```python
from build123d import *

# Parameters (mm, degrees)
BOSS_EXTRUDE1_DEPTH = 20
SKETCH1_3_R         = 40
SKETCH1_3_R_2       = 25
BOSS_EXTRUDE2_DEPTH = 40
BOSS_EXTRUDE3_DEPTH = 70


with BuildPart() as part:
    # Sketch1 → Boss-Extrude1 (new body)
    with BuildSketch(Plane(origin=(0, 0, 0), x_dir=(1, 0, 0), z_dir=(0, 1, 0))):
        with BuildLine():
            ThreePointArc((-47.892857143, -57.717191847), (-25.457912439, -70.547109751), (0, -75))
            Line((0, -75), (0, -60))
            ThreePointArc((0, -60), (-60, 0), (0, 60))
            Line((0, 60), (0, 75))
            ThreePointArc((0, 75), (-25.457912439, 70.547109751), (-47.892857143, 57.717191847))
            ThreePointArc((-47.892857143, 57.717191847), (-91.104177178, 36.827906099), (-139.071428571, 38.478127898))
            ThreePointArc((-139.071428571, 38.478127898), (-118.084934144, 24.112830017), (-110, 0))
            ThreePointArc((-110, 0), (-118.084934144, -24.112830017), (-139.071428571, -38.478127898))
            ThreePointArc((-139.071428571, -38.478127898), (-91.104177178, -36.827906099), (-47.892857143, -57.717191847))
        make_face()
        with BuildLine():
            Line((0, -60), (0, -75))
            ThreePointArc((0, -75), (25.457912439, -70.547109751), (47.892857143, -57.717191847))
            ThreePointArc((47.892857143, -57.717191847), (91.104177178, -36.827906099), (139.071428571, -38.478127898))
            ThreePointArc((139.071428571, -38.478127898), (110, 0), (139.071428571, 38.478127898))
            ThreePointArc((139.071428571, 38.478127898), (91.104177178, 36.827906099), (47.892857143, 57.717191847))
            ThreePointArc((47.892857143, 57.717191847), (25.457912439, 70.547109751), (0, 75))
            Line((0, 75), (0, 60))
            ThreePointArc((0, 60), (42.426406871, 42.426406871), (60, 0))
            ThreePointArc((60, 0), (42.426406871, -42.426406871), (0, -60))
        make_face()
    extrude(amount=BOSS_EXTRUDE1_DEPTH)

    # Sketch1_3 → Boss-Extrude2 (add)
    # profile 1 of 2: a face of its own
    with BuildSketch(Plane(origin=(0, 0, 0), x_dir=(1, 0, 0), z_dir=(0, 1, 0))):
        with Locations(Location((-150, 0, 0), (0, 0, 74.144374523))):
            Circle(SKETCH1_3_R)
        with Locations(Location((-150, 0, 0), (0, 0, 270))):
            Circle(SKETCH1_3_R_2, mode=Mode.SUBTRACT)
    # profile 2 of 2: a face of its own
    with BuildSketch(Plane(origin=(0, 0, 0), x_dir=(1, 0, 0), z_dir=(0, 1, 0))):
        with Locations(Location((150, 0, 0), (0, 0, 105.855625477))):
            Circle(SKETCH1_3_R)
        with Locations(Location((150, 0, 0), (0, 0, 270))):
            Circle(SKETCH1_3_R_2, mode=Mode.SUBTRACT)
    extrude(amount=BOSS_EXTRUDE2_DEPTH)

    # Sketch1_4 → Boss-Extrude3 (add)
    with BuildSketch(Plane(origin=(0, 0, 0), x_dir=(1, 0, 0), z_dir=(0, 1, 0))):
        with BuildLine():
            ThreePointArc((0, 60), (-60, 0), (0, -60))
            Line((0, -60), (0, -50))
            ThreePointArc((0, -50), (-50, 0), (0, 50))
            Line((0, 50), (0, 60))
        make_face()
        with BuildLine():
            Line((0, -50), (0, -60))
            ThreePointArc((0, -60), (42.426406871, -42.426406871), (60, 0))
            ThreePointArc((60, 0), (42.426406871, 42.426406871), (0, 60))
            Line((0, 60), (0, 50))
            ThreePointArc((0, 50), (35.355339059, 35.355339059), (50, 0))
            ThreePointArc((50, 0), (35.355339059, -35.355339059), (0, -50))
        make_face()
    extrude(amount=BOSS_EXTRUDE3_DEPTH)


solid = part.part
```
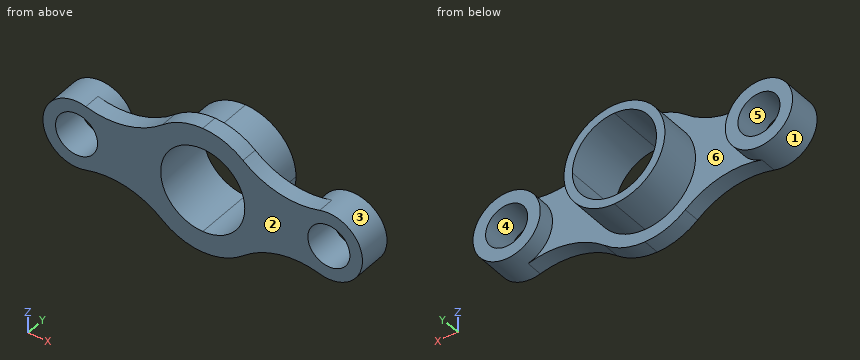
Design review of the part built by this model. Coordinates are the model's own, in mm. Face numbers are marked on the shaded views. A direction names the side the tool comes from. Coordinates: 2 decimals unless noted, no trailing zeros. Order: outer loops, then holes, each group sorted by start corner. A loop starts at its lowest first (then second) coordinate and runs counter-clockwise, first axis right, second up. Notation, with made-up numbers: M 80,23.5 L 91,23.5 A6 cw 91,28.5 Z; hole C 51.25,45.5 d4. An arc over 180 degrees is marked long. Answer as a JSON object with one key per item and string values. Group by question number.
1) Add section B-B, the plane x = -150. Write out the cut boundary in (y, z), then the cut area to 3 significant figures.
2) Add section C-C, the plane z = 10.5. Write out the cut boundary in (x, y), then the cut area to 3 significant figures.
3) Tool access review of the marked faces 1 and 2: name each direction out of +Z, -Z, +X, -X, +Y, -Y from which nothing blocks a thin tool from reaching the whole face with its end or side.
4) For pin 1 (12 mm diameter, centred on x = -87, z = 10, fed in from +Y); pin 2 (6 mm diameter, centred on y = 38, z = -7.5, fed in from +X); pin 3 (2 mm diameter, centred on x = 55.5, y = 58.5, fed in from -Z), all flat-tipped, find the tip position at first contact; note any pin that passes through.
5) Mouldability with a two-part tool opening along Z and no side actions: class the marked faces 3, 4, 5 and 6 as pulls with the +Z half, pulls with the -Z half, needs draft (parallel to the pull), parting line crosses it, or undercut.
6) Add section A-A, the plane y = 25. Write out the cut boundary in (x, z), then the cut area to 3 significant figures.
7) Wall thickness on L1, parallel to X at y = 15, z = 0; L2, parallel to Y at x = -102, z = 13.5; L3, parallel to Z at x = 22, y = 56.5: over which ranges is each line inside the solid? List them lowest first.
8) Add section D-D, the plane x = 120.5. Write out the cut boundary in (y, z), then the cut area to 3 significant figures.
Computed values:
{
 "1": {"outline": "M 0,-40 L 40,-40 L 40,-25 L 0,-25 Z; M 0,25 L 40,25 L 40,40 L 0,40 Z", "area": "1,200 mm^2"},
 "2": {"outline": "M -188.6,0 L -172.69,0 L -172.69,40 L -188.6,40 Z; M -127.31,0 L -48.89,0 L -48.89,70 L -59.07,70 L -59.07,20 L -111.4,20 L -111.4,40 L -127.31,40 Z; M 48.89,0 L 127.31,0 L 127.31,40 L 111.4,40 L 111.4,20 L 59.07,20 L 59.07,70 L 48.89,70 Z; M 172.69,0 L 188.6,0 L 188.6,40 L 172.69,40 Z", "area": "6,070 mm^2"},
 "3": {"face 1": "+Y", "face 2": "+Z, -Z, +X, -X, -Y"},
 "4": {"pin 1": "stops at y = 20", "pin 2": "stops at x = 189.75", "pin 3": "stops at z = -25.09"},
 "5": {"face 3": "parting line crosses it", "face 4": "undercut", "face 5": "undercut", "face 6": "needs draft"},
 "6": {"outline": "C -150,0 d80; C 0,0 d120; C 150,0 d80; hole C -150,0 d50; hole C 0,0 d100; hole C 150,0 d50", "area": "9,580 mm^2"},
 "7": {"L1": "x = -190 to -175, -125 to -50, 50 to 125, 175 to 190", "L2": "y = 0 to 20", "L3": "z = -55.82 to -44.9, 44.9 to 55.82"},
 "8": {"outline": "M 0,-35.06 L 20,-35.06 L 20,-27.01 L 40,-27.01 L 40,27.01 L 20,27.01 L 20,35.06 L 0,35.06 Z", "area": "2,480 mm^2"}
}
